```python
from build123d import *

# Parameters (mm, degrees)
F1_DEPTH  = 15
F2_R      = 2
F4_DEPTH  = 25
F5_DEPTH  = 4
F6_DEPTH  = 25
F8_DEPTH  = 25
F9_DEPTH  = 4
F10_DEPTH = 25


with BuildPart() as f1:
    # F0 (on Front) → F1 (new body)
    with BuildSketch(Plane.XZ):
        with BuildLine():
            ThreePointArc((-23.1304047869, 0.0265709655), (1.8676618749, 25.0246376273), (26.8657285366, 0.0265709655))
            Line((26.8657285366, 0.0265709655), (38.8657285366, 0.0265709655))
            Line((38.8657285366, 0.0265709655), (38.8657285366, 7.0265709655))
            Line((38.8657285366, 7.0265709655), (30.8657285366, 7.0265709655))
            ThreePointArc((30.8657285366, 7.0265709655), (1.8676618749, 30.1297350471), (-27.1304047869, 7.0265709655))
            Line((-27.1304047869, 7.0265709655), (-35.1304047869, 7.0265709655))
            Line((-35.1304047869, 7.0265709655), (-35.1304047869, 0.0265709655))
            Line((-35.1304047869, 0.0265709655), (-23.1304047869, 0.0265709655))
        make_face()
    extrude(amount=F1_DEPTH)

    # F2
    f2_edges = [f1.edges().sort_by_distance(p)[0] for p in [
        (1.867662, -15, 30.129735),
        (34.865729, -15, 7.026571),
        (38.865729, -15, 3.526571),
        (38.865729, -7.5, 7.026571),
        (-31.130405, -15, 7.026571),
        (-35.130405, -15, 3.526571),
        (-35.130405, -7.5, 7.026571),
        (1.867662, 0, 30.129735),
        (-31.130405, 0, 7.026571),
        (-35.130405, 0, 3.526571),
        (34.865729, 0, 7.026571),
        (38.865729, 0, 3.526571),
    ]]
    fillet(f2_edges, radius=F2_R)

    # F3 (on face) → F4 (cut)
    with BuildSketch(Plane.XY.offset(7.0265709655)):
        with BuildLine():
            ThreePointArc((36.8657285366, -7.7325071808), (36.875896312, -7.6164511554), (36.8792894082, -7.5))
            ThreePointArc((36.8792894082, -7.5), (36.875896312, -7.3835488446), (36.8657285366, -7.2674928192))
            Line((36.8657285366, -7.2674928192), (36.8657285366, -7.7325071808))
        make_face()
    extrude(amount=-F4_DEPTH, mode=Mode.SUBTRACT)

    # F3 (on face) → F5 (cut)
    with BuildSketch(Plane.XY.offset(7.0265709655)):
        with BuildLine():
            ThreePointArc((36.8657285366, -7.7325071808), (32.8792894082, -7.5), (36.8657285366, -7.2674928192))
            Line((36.8657285366, -7.2674928192), (36.8657285366, -4.6048032856))
            Line((36.8657285366, -4.6048032856), (34.8714804252, -3.45855566))
            Line((34.8714804252, -3.45855566), (31.3753914503, -5.4860406077))
            Line((31.3753914503, -5.4860406077), (31.3832004333, -9.5274849477))
            Line((31.3832004333, -9.5274849477), (34.8870983913, -11.54144434))
            Line((34.8870983913, -11.54144434), (36.8657285366, -10.3939784529))
            Line((36.8657285366, -10.3939784529), (36.8657285366, -7.7325071808))
        make_face()
        with BuildLine():
            ThreePointArc((36.8657285366, -7.2674928192), (36.875896312, -7.3835488446), (36.8792894082, -7.5))
            ThreePointArc((36.8792894082, -7.5), (36.875896312, -7.6164511554), (36.8657285366, -7.7325071808))
            Line((36.8657285366, -7.7325071808), (36.8657285366, -10.3939784529))
            Line((36.8657285366, -10.3939784529), (38.3831873661, -9.5139593923))
            Line((38.3831873661, -9.5139593923), (38.3753783831, -5.4725150523))
            Line((38.3753783831, -5.4725150523), (36.8657285366, -4.6048032856))
            Line((36.8657285366, -4.6048032856), (36.8657285366, -7.2674928192))
        make_face()
    extrude(amount=-F5_DEPTH, mode=Mode.SUBTRACT)

    # F3 (on face) → F6 (cut)
    with BuildSketch(Plane.XY.offset(7.0265709655)):
        with BuildLine():
            Line((36.8657285366, -7.7325071808), (36.8657285366, -7.2674928192))
            ThreePointArc((36.8657285366, -7.2674928192), (32.8792894082, -7.5), (36.8657285366, -7.7325071808))
        make_face()
    extrude(amount=-F6_DEPTH, mode=Mode.SUBTRACT)

    # F7 (on face) → F8 (cut)
    with BuildSketch(Plane.XY.offset(7.0265709655)):
        with BuildLine():
            ThreePointArc((-33.1304047869, -7.74764379), (-31.0207948898, -9.4935798639), (-29.1461082168, -7.4975095821))
            ThreePointArc((-29.1461082168, -7.4975095821), (-31.0207948898, -5.5014393002), (-33.1304047869, -7.2473753741))
            Line((-33.1304047869, -7.2473753741), (-33.1304047869, -7.74764379))
        make_face()
    extrude(amount=-F8_DEPTH, mode=Mode.SUBTRACT)

    # F7 (on face) → F9 (cut)
    with BuildSketch(Plane.XY.offset(7.0265709655)):
        with BuildLine():
            ThreePointArc((-33.1304047869, -7.74764379), (-33.1461082168, -7.4975095821), (-33.1304047869, -7.2473753741))
            Line((-33.1304047869, -7.2473753741), (-33.1304047869, -4.6022885965))
            Line((-33.1304047869, -4.6022885965), (-34.6500061748, -5.4835501898))
            Line((-34.6500061748, -5.4835501898), (-34.6421971917, -9.5249945298))
            Line((-34.6421971917, -9.5249945298), (-33.1304047869, -10.3939377894))
            Line((-33.1304047869, -10.3939377894), (-33.1304047869, -7.74764379))
        make_face()
        with BuildLine():
            ThreePointArc((-33.1304047869, -7.2473753741), (-31.0207948898, -5.5014393002), (-29.1461082168, -7.4975095821))
            ThreePointArc((-29.1461082168, -7.4975095821), (-31.0207948898, -9.4935798639), (-33.1304047869, -7.74764379))
            Line((-33.1304047869, -7.74764379), (-33.1304047869, -10.3939377894))
            Line((-33.1304047869, -10.3939377894), (-31.1382992338, -11.5389539221))
            Line((-31.1382992338, -11.5389539221), (-27.6422102589, -9.5114689744))
            Line((-27.6422102589, -9.5114689744), (-27.650019242, -5.4700246344))
            Line((-27.650019242, -5.4700246344), (-31.1539171999, -3.4560652421))
            Line((-31.1539171999, -3.4560652421), (-33.1304047869, -4.6022885965))
            Line((-33.1304047869, -4.6022885965), (-33.1304047869, -7.2473753741))
        make_face()
    extrude(amount=-F9_DEPTH, mode=Mode.SUBTRACT)

    # F7 (on face) → F10 (cut)
    with BuildSketch(Plane.XY.offset(7.0265709655)):
        with BuildLine():
            Line((-33.1304047869, -7.74764379), (-33.1304047869, -7.2473753741))
            ThreePointArc((-33.1304047869, -7.2473753741), (-33.1461082168, -7.4975095821), (-33.1304047869, -7.74764379))
        make_face()
    extrude(amount=-F10_DEPTH, mode=Mode.SUBTRACT)


solid = f1.part
```
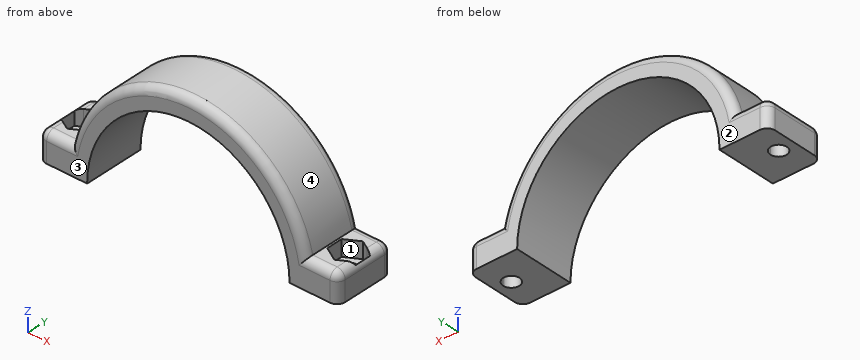
Could you check a few things on this model? Use its own coordinates, in mm. Face numbers are marked on the shaded views. Give positions to 0.01 mm unless a question says otherwise; leave off trailing zeros. Answer in a Markdown table with one row per item. Add a question column.
Q1. We'd pull the mould along Y, two halves only. Please class the marked faces 1, 2, 3 and 4: +Y half, -Y half, draft (parallel to the pull), parting line (faces both ways), or undercut.
Q2. For pin 1 (10 mm diameter, centred on x = -8.5, z = 13, fed in from -Y); pin 2 (3.5 mm diameter, centred on x = -32.5, y = -8.5, fed in from +Z); pin 3 (1.5 mm diameter, centred on y = -4.5, z = 19.5, fed in from +X); pin 4 (5 mm diameter, centred on y = -9, z = 14, fed in from -X), each with a flat end and sliding along its axis, tell me the tip position at first contact or that it passes through.
Q3. Please list where these lines run through material, in increasing order: L1, parallel to X at y = -7.5, z = 2.4; L2, parallel to X at y = -4, z = 22; L3, parallel to Y at x = -28.5, z = 5.5. Write a range as from..to.
The answers:
| question | item | result |
|---|---|---|
| 1 | face 1 | undercut |
| 1 | face 2 | +Y half |
| 1 | face 3 | -Y half |
| 1 | face 4 | draft |
| 2 | pin 1 | passes through |
| 2 | pin 2 | stops at z = 3.03 |
| 2 | pin 3 | stops at x = 25.27 |
| 2 | pin 4 | stops at x = -25.73 |
| 3 | L1 | x = -35.13..-33.15, -29.15..-23.02, 26.75..32.88, 36.88..38.87 |
| 3 | L2 | x = -18.57..-10.05, 13.79..22.3 |
| 3 | L3 | y = -14.94..-10.01, -4.98..-0.06 |
